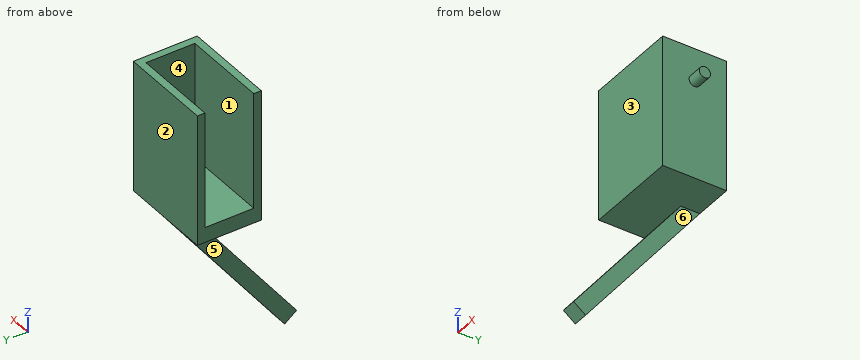
```python
from build123d import *

# Parameters (mm, degrees)
SKETCH2_W           = 25
SKETCH2_H           = 17
BOSS_EXTRUDE1_DEPTH = 35
BOSS_EXTRUDE2_START = -12.5
BOSS_EXTRUDE2_DEPTH = 2
SKETCH4_W           = 26
SKETCH4_H           = 10
CUT_EXTRUDE1_DEPTH  = 10
SKETCH5_W           = 23
SKETCH5_H           = 13
CUT_EXTRUDE2_DEPTH  = 31
SKETCH6_R           = 1.5
BOSS_EXTRUDE4_DEPTH = 4


with BuildPart() as part:
    # Sketch2 → Boss-Extrude1 (new body)
    with BuildSketch(Plane.XY):
        with Locations((0.358490566, 2.41509434)):
            Rectangle(SKETCH2_W, SKETCH2_H)
    extrude(amount=BOSS_EXTRUDE1_DEPTH)

    # Sketch3 → Boss-Extrude2 (add, symmetric)
    with BuildSketch(Plane.ZY.offset(12.141509434).offset(BOSS_EXTRUDE2_START)):
        Polygon((0, 10.91509434), (-39.708579083, -19.469585142), (-37.277804725, -22.646271469), (0, 5.878399383), align=None)
    extrude(amount=BOSS_EXTRUDE2_DEPTH, both=True)

    # Sketch4 → Cut-Extrude1 (cut)
    with BuildSketch(Plane.ZY.offset(12.141509434)):
        with Locations((22, 2.41509434)):
            Rectangle(SKETCH4_W, SKETCH4_H)
    extrude(amount=-CUT_EXTRUDE1_DEPTH, mode=Mode.SUBTRACT)

    # Sketch5 → Cut-Extrude2 (cut)
    with BuildSketch(Plane.XY.offset(35)):
        with Locations((-0.641509434, 2.41509434)):
            Rectangle(SKETCH5_W, SKETCH5_H)
    extrude(amount=-CUT_EXTRUDE2_DEPTH, mode=Mode.SUBTRACT)

    # Sketch6 → Boss-Extrude4 (add)
    with BuildSketch(Plane(origin=(12.858490566, 0, 0), x_dir=(0, 0, -1), z_dir=(1, 0, 0))):
        with Locations(Location((-26.251622056, 2.426562122, 0), (0, 0, 90))):
            Circle(SKETCH6_R)
    extrude(amount=BOSS_EXTRUDE4_DEPTH)


solid = part.part
```
The model under review builds one solid part; all positions refer to its coordinate system, in mm. Face numbers are marked on the shaded views. A direction names the side the tool comes from. Round coordinates to 2 decimals unless told otherwise and drop trailing zeros. Loops run counter-clockwise (first coordinate to the right, second up) from the corner with the lowest first, then second, coordinate; pieces in that order, holes last. Notation, with made-up numbers: (88.25, -28.75) -> (129.25, -28.75) arc R5 cw to (129.25, -24.75) -> close; hole circle Ø8 at (-8.75, -38). An arc over 180 degrees is marked (long way). Answer as a JSON object with one key per item and string values. Group by question number.
1) Mouldability with a two-part tool opening along Y and no side actions: class the marked faces 1, 2 and 3 as released by +Y, released by -Y, zero draft, split by the parting line, or undercut.
2) We need section A-A on x = -5. Write out the cut boundary in (y, z), then the cut area to 3 significant figures.
3) For pin 1 Ø6.5 at (y, z) = (2.5, 24) entering from -X; pin 2 Ø7 at (x, z) = (-5, 21.5) entering from -Y; pin 3 Ø13.5 at (x, y) = (-0.5, 6) entering from -Z, all flat-tipped, find the tip position at first contact; note any pin that passes through.
4) For line 1 (Y direction, x = 6, z = 17); line 2 (Z direction, x = -4, y = -1); line 3 (Z direction, x = 2.75, y = -6), list the stretches that pass through material, from the lowest coordinate up. Write a range as [from, to].
5) We need section B-B on z = 13. Write out the cut boundary in (x, y).
6) We need section C-C on y = -2.5. Write out the cut boundary in (x, z).
7) We need section D-D on x = 0.75. Write out the cut boundary in (y, z), then the cut area to 3 significant figures.
8) For the marked faces 4, 5 and 6, list the 3-axis set-ups (+Z, -Z, +X, -X, +Y, -Y) from which the entire face can be reached by the end or side of a thin tool; tool diameter is ignored.
Result set:
{
 "1": {"face 1": "undercut", "face 2": "released by +Y", "face 3": "released by -Y"},
 "2": {"outline": "(-6.08, 0) -> (10.92, 0) -> (10.92, 35) -> (8.92, 35) -> (8.92, 4) -> (-4.08, 4) -> (-4.08, 35) -> (-6.08, 35) -> close", "area": "192 mm²"},
 "3": {"pin 1": "x = 10.86", "pin 2": "y = -6.08", "pin 3": "z = -15.24"},
 "4": {"line 1": "[-6.08, -4.08], [8.92, 10.92]", "line 2": "[0, 4]", "line 3": "[0, 35]"},
 "5": {"outline": "(-12.14, -6.08) -> (12.86, -6.08) -> (12.86, 10.92) -> (-12.14, 10.92) -> (-12.14, 8.92) -> (10.86, 8.92) -> (10.86, -4.08) -> (-12.14, -4.08) -> close"},
 "6": {"outline": "(-12.14, 0) -> (12.86, 0) -> (12.86, 35) -> (10.86, 35) -> (10.86, 4) -> (-12.14, 4) -> close; (-1.64, -17.53) -> (2.36, -17.53) -> (2.36, -10.95) -> (-1.64, -10.95) -> close"},
 "7": {"outline": "(-22.65, -37.28) -> (-19.47, -39.71) -> (10.92, 0) -> (10.92, 35) -> (8.92, 35) -> (8.92, 4) -> (-4.08, 4) -> (-4.08, 35) -> (-6.08, 35) -> (-6.08, 0) -> (5.88, 0) -> close", "area": "386 mm²"},
 "8": {"face 4": "+Z, -X", "face 5": "-Z, -X, +Y, -Y", "face 6": "-Z, +X, +Y, -Y"}
}
